```python
from build123d import *

# Parameters (mm, degrees)
F1_DEPTH = 4.064


with BuildPart() as f1:
    # F0 (on Top) → F1 (new body)
    with BuildSketch(Plane.XY):
        with BuildLine():
            ThreePointArc((-3.0053685298, -2.921), (-3.860465775, 1.6313445375), (0, 4.191))
            Line((0, 4.191), (11.9885578365, 4.191))
            ThreePointArc((11.9885578365, 4.191), (-12.6827588318, -0.6615348929), (12.3595209859, -2.921))
            Line((12.3595209859, -2.921), (3.0053685298, -2.921))
            ThreePointArc((3.0053685298, -2.921), (0, -4.191), (-3.0053685298, -2.921))
        make_face()
        with BuildLine():
            ThreePointArc((0, 4.191), (2.96348452, 2.96348452), (4.191, 0))
            ThreePointArc((4.191, 0), (3.883296313, -1.5762267431), (3.0053685298, -2.921))
            Line((3.0053685298, -2.921), (12.3595209859, -2.921))
            ThreePointArc((12.3595209859, -2.921), (12.6145930676, -1.4703882956), (12.7, 0))
            ThreePointArc((12.7, 0), (12.5208762578, 2.1254782375), (11.9885578365, 4.191))
            Line((11.9885578365, 4.191), (0, 4.191))
        make_face()
        with BuildLine():
            ThreePointArc((-3.0053685298, -2.921), (0, -4.191), (3.0053685298, -2.921))
            Line((3.0053685298, -2.921), (-3.0053685298, -2.921))
        make_face()
    extrude(amount=F1_DEPTH)


solid = f1.part
```
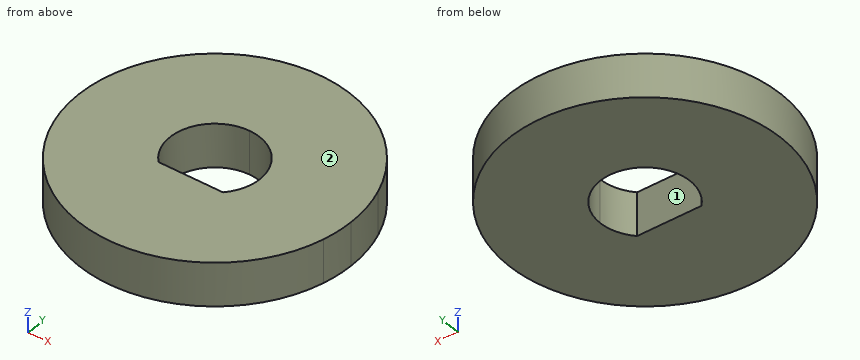
Design review of the part built by this model. Coordinates are the model's own, in mm. Face numbers are marked on the shaded views. Round coordinates to 2 decimals unless told otherwise and drop trailing zeros. Write each loop counter-clockwise with the first axis right and the second up, starting at its lowest first coordinate (ties: lowest second). Pieces come first, ordered by that corner, then holes. Notation, with made-up numbers: (43, 88) -> (100, 88) arc R26 ccw to (100, 104) -> close; hole circle Ø10 at (76, 58). An arc over 180 degrees is marked (long way). Write item = value, one per line. Start each with the question number.
1) Take a section at B-B, the plane y = 11. State the section outline as (x, z) points, plus the area to 3 significant figures.
2) Wall thickness on probe 1 along Y at (x, z) = (-1.5, 0.9); probe 2 along X at (y, z) = (-2.5, 3.55); probe 3 along Y at (x, z) = (-1, 1.65): over which ranges is each line inside the solid? List them lowest first. Write a range as from..to.
3) Take a section at A-A, the plane z = 2.75. State the section outline as (x, y) points.
4) Take a section at C-C, the plane x = -5.5. State the section outline as (y, z) points.
5) Clearance check with flat-ended pins moving along their axes: pin 1 (1 mm diameter, centred on y = 4, z = 2, fed in from +X); pin 2 (1 mm diameter, centred on x = -4.5, z = 2, fed in from -Y). State where each tip first meets the part, or that it passes through.
6) Mouldability with a two-part tool opening along X and no side actions: class the marked faces 1 and 2 as +X half, -X half, draft (parallel to the pull), parting line (faces both ways), or undercut.
Results list:
q1.outline = (-6.35, 0) -> (6.35, 0) -> (6.35, 4.06) -> (-6.35, 4.06) -> close
q1.area = 51.6 mm²
q2.probe_1 = -12.61..-2.92, 3.91..12.61
q2.probe_2 = -12.45..-3.36, 3.36..12.45
q2.probe_3 = -12.66..-2.92, 4.07..12.66
q3.outline = circle Ø25.4 at (0, 0); hole (-3.01, -2.92) -> (3.01, -2.92) arc R4.19 ccw (long way) to start
q4.outline = (-11.45, 0) -> (11.45, 0) -> (11.45, 4.06) -> (-11.45, 4.06) -> close
q5.pin_1 = 12.21
q5.pin_2 = -12.05
q6.face_1 = undercut
q6.face_2 = draft
